Could you check a few things on this model? Use its own coordinates, in mm. Give positions to 0.01 mm unless a question says otherwise; leave off trailing zeros. Write each loop counter-clockwise with the first axis right and the second up, starting at its lowest first coordinate (ties: lowest second). Pieces come first, ordered by that corner, then holes. Notation, with made-up numbers: (-13.5, 88.25) -> (43.5, 88.25) arc R29 ccw to (43.5, 121.25) -> close; hole circle Ø5 at (46.5, -8.75). An arc over 180 degrees is marked (long way). Write item = value, one per line. Start each with the question number.
```python
from build123d import *

# Parameters (mm, degrees)
SKETCH2_R           = 63.5
BOSS_EXTRUDE1_DEPTH = 15
SKETCH3_R           = 1.45
CUT_EXTRUDE1_DEPTH  = 92.046691318
FILLET2_R           = 0.5


with BuildPart() as part:
    # Sketch2 → Boss-Extrude1 (new body)
    with BuildSketch(Plane(origin=(0, 0, 0), x_dir=(1, 0, 0), z_dir=(0, 1, 0))):
        with Locations(Location((0, 0, 0), (0, 0, 270))):
            Circle(SKETCH2_R)
    extrude(amount=BOSS_EXTRUDE1_DEPTH)

    # Sketch3 → Cut-Extrude1 (cut, through all)
    with BuildSketch(Plane(origin=(0, 15, 0), x_dir=(1, 0, 0), z_dir=(0, 1, 0))):
        with Locations(Location((0, 8, 0), (0, 0, 270))):
            Circle(SKETCH3_R)
        with Locations(Location((8, 0, 0), (0, 0, 270))):
            Circle(SKETCH3_R)
        with Locations(Location((0, -8, 0), (0, 0, 270))):
            Circle(SKETCH3_R)
        with Locations(Location((-8, 0, 0), (0, 0, 270))):
            Circle(SKETCH3_R)
    extrude(amount=-CUT_EXTRUDE1_DEPTH, mode=Mode.SUBTRACT)

    # Fillet2
    fillet2_edges = [part.edges().sort_by_distance(p)[0] for p in [
        (0, 0, -63.5),
        (0, 15, -63.5),
    ]]
    fillet(fillet2_edges, radius=FILLET2_R)


solid = part.part
```
(1) If I drill on line 1 along X through (y, z) = (5.75, 0); line 2 along Z through (x, y) = (-1, 1.25); line 3 along X through (y, z) = (11.25, -8), over which ranges is the centre line in solid material (lowest first)? Write a range as from..to.
(2) I'm going to push flat-ended pins straight in: pin 1 (1.5 mm diameter, centred on x = -18.5, y = 7.5, fed in from -Z); pin 2 (3 mm diameter, centred on y = 10, z = -3.5, fed in from +X); pin 3 (5 mm diameter, centred on y = 3, z = 36, fed in from +X); pin 4 (2.5 mm diameter, centred on x = -8, z = 0, fed in from -Y). Where does each tip first touch, or does it pass through?
(3) We'd pull the mould along Z, two halves only. Please class faces 1 (the flat face through (1, 15, -1)), 2 (the cylindrical face through (-61.99, 7.4, -13.77)), 3 (the cylindrical face through (6.584, 7.605, -0.314)): released by +Z, released by -Z, zero draft, split by the parting line, or undercut.
(4) Imagine slicing it at A-A (x = 0). Please give me the cut outline in (y, z).
(5) Imagine slicing it at C-C (y = 5.25). Please give me the cut outline in (x, z), then the cut area to 3 significant figures.
(6) Imagine slicing it at B-B (z = 0). Please give me the cut outline in (x, y), then the cut area to 3 significant figures.
Answers below:
q1.line_1 = -63.5..-9.45, -6.55..6.55, 9.45..63.5
q1.line_2 = -63.49..-9.05, -6.95..6.95, 9.05..63.49
q1.line_3 = -62.99..-1.45, 1.45..62.99
q2.pin_1 = -60.97
q2.pin_2 = 63.47
q2.pin_3 = 53.94
q2.pin_4 = through
q3.face_1 = zero draft
q3.face_2 = split by the parting line
q3.face_3 = undercut
q4.outline = (0, -63) arc R0.5 ccw to (0.5, -63.5) -> (14.5, -63.5) arc R0.5 ccw to (15, -63) -> (15, -9.45) -> (0, -9.45) -> close; (0, -6.55) -> (15, -6.55) -> (15, 6.55) -> (0, 6.55) -> close; (0, 9.45) -> (15, 9.45) -> (15, 63) arc R0.5 ccw to (14.5, 63.5) -> (0.5, 63.5) arc R0.5 ccw to (0, 63) -> close
q5.outline = circle Ø127 at (0, 0); hole circle Ø2.9 at (-8, 0); hole circle Ø2.9 at (0, -8); hole circle Ø2.9 at (0, 8); hole circle Ø2.9 at (8, 0)
q5.area = 12,600 mm^2
q6.outline = (-63.5, 0.5) arc R0.5 ccw to (-63, 0) -> (-9.45, 0) -> (-9.45, 15) -> (-63, 15) arc R0.5 ccw to (-63.5, 14.5) -> close; (-6.55, 0) -> (6.55, 0) -> (6.55, 15) -> (-6.55, 15) -> close; (9.45, 0) -> (63, 0) arc R0.5 ccw to (63.5, 0.5) -> (63.5, 14.5) arc R0.5 ccw to (63, 15) -> (9.45, 15) -> close
q6.area = 1,820 mm^2
